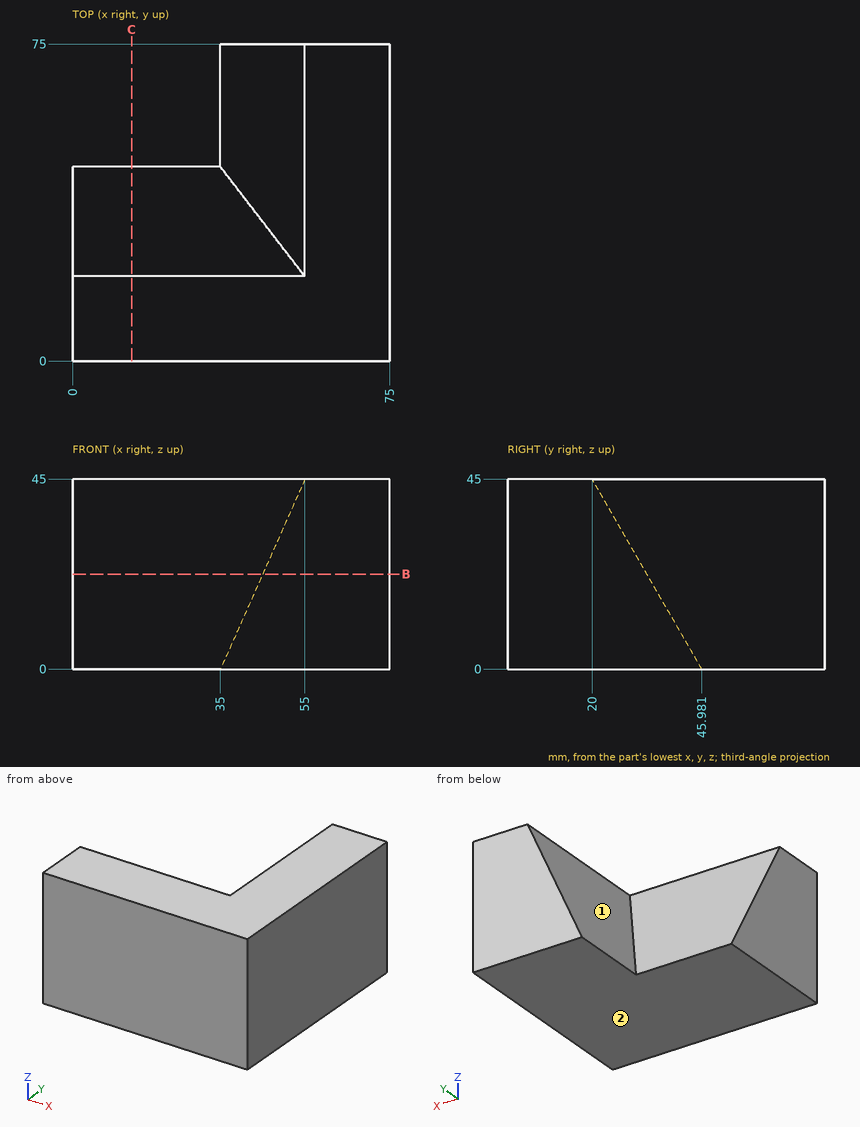
For this review, use the dimensioned drawing (mm, ordinates from the lowest corner) and the shaded views. A direction names the side the tool comes from. Round coordinates to 2 decimals unless told otherwise and drop trailing zeros. Order: outer loops, then holes, each group sorted by start corner. A loop starts at its lowest first (then second) coordinate and runs counter-clockwise, first axis right, second up. Notation, with made-up numbers: (-26, 4.25) -> (28, 4.25) arc R20 cw to (28, 37.25) -> close; hole circle Ø1 at (-33.5, 66.25). An arc over 180 degrees is marked (long way). One line per item, written item: value. Start each with the question number.
Q1. Wall thickness on line 1 (X direction, y = 37.5, z = 22.5); line 2 (Z direction, x = 27, y = 41) (1 decimal); line 3 (X direction, y = 69, z = 42): over which ranges is each line inside the solid? List them lowest first.
Q2. Machinability: for the marked faces 1 and 2, which of the approach directions +Z, -Z, +X, -X, +Y, -Y give a long, thin tool a straight path to every point of the face, cutting with its end or side? Answer none if there is none.
Q3. Take a section at B-B (z = 22.5). Write out the cut boundary in (x, y), and give its area (3 significant figures).
Q4. Take a section at C-C (x = 14). Write out the cut boundary in (y, z).
Q5. Clearance check with flat-ended pins moving along their axes: pin 1 Ø3 at (x, y) = (37, 44.5) entering from +Z (1 decimal); pin 2 Ø1.5 at (x, z) = (24.5, 22.5) entering from +Y; pin 3 Ø6 at (y, z) = (49, 22.5) entering from -X. State where each tip first meets the part, or that it passes through.
Reported:
1. line 1: x = 45 to 75
1. line 2: z = 0 to 8.6
1. line 3: x = 53.67 to 75
2. face 1: +Z, -X, +Y
2. face 2: -Z, +X, -X, +Y, -Y
3. outline: (0, 0) -> (75, 0) -> (75, 75) -> (45, 75) -> (45, 32.99) -> (0, 32.99) -> close
3. area: 3,730 mm2
4. outline: (0, 0) -> (45.98, 0) -> (20, 45) -> (0, 45) -> close
5. pin 1: stops at z = 7.9
5. pin 2: stops at y = 33.42
5. pin 3: stops at x = 43.67
